Geometry check sheet. Reference: the model listing, model coordinates, mm. Face numbers are marked on the shaded views. A direction names the side the tool comes from. Coordinates: 2 decimals unless noted, no trailing zeros. Loops run counter-clockwise (first coordinate to the right, second up) from the corner with the lowest first, then second, coordinate; pieces in that order, holes last. Notation, with made-up numbers: (51, 73) - (100, 73) arc R36 cw to (100, 107) - close; hole circle Ø5 at (11, -7). An arc over 180 degrees is marked (long way). One line per item, written item: value.
from build123d import *

# Parameters (mm, degrees)
SKETCH1_R                    = 1.1303
BASE_DEPTH                   = 1.5
SKETCH1_4_W                  = 14.75
SKETCH1_4_H                  = 2
BOTTOM_WALLS_DEPTH           = 11
F_4_40_CLOSE_FIT_CLEAR_REACH = 41.1
SKETCH2_R                    = 1.4732
SKETCH1_8_W                  = 2
SKETCH1_8_H                  = 30.5
MIDDLE_WALLS_DEPTH           = 7
ROOF_START                   = 7
ROOF_OUTLINE_W               = 9.75
ROOF_OUTLINE_H               = 34.5
ROOF_DEPTH                   = 1
SKETCH1_5_W                  = 1.425
SKETCH1_5_H                  = 2.85
CUT_EXTRUDE2_DEPTH           = 8
FILLET1_R                    = 0.25


# Read off the part's stored shape, not the designer's step: Roof
with BuildPart() as part:
    # Sketch1 → Base (new body)
    with BuildSketch(Plane(origin=(0, 0, 0), x_dir=(1, 0, 0), z_dir=(0, 1, 0))):
        Polygon((5, -2), (14.75, -2), (14.75, 0), (0, 0), (0, -34.5), (14.75, -34.5), (14.75, -32.5), (5, -32.5), align=None)
        with Locations(Location((2.75, -7.25, 0), (0, 0, 270))):
            Circle(SKETCH1_R, mode=Mode.SUBTRACT)
        with Locations(Location((2.75, -27.25, 0), (0, 0, 270))):
            Circle(SKETCH1_R, mode=Mode.SUBTRACT)
    extrude(amount=BASE_DEPTH)

    # Sketch1<4> → Bottom Walls (add)
    with BuildSketch(Plane(origin=(0, 0, 0), x_dir=(1, 0, 0), z_dir=(0, 1, 0))):
        with Locations((7.375, -1)):
            Rectangle(SKETCH1_4_W, SKETCH1_4_H)
        with Locations((7.375, -33.5)):
            Rectangle(SKETCH1_4_W, SKETCH1_4_H)
    extrude(amount=-BOTTOM_WALLS_DEPTH)

    # 4-40_Close_fit Clear: up to this face of the body (flat: up to its plane)
    f_4_40_close_fit_clear_end = Plane(part.part.faces().sort_by_distance((7.375, -4.75, 0))[0])
    # Sketch2 → 4-40_Close_fit Clear (cut, up to the picked face)
    with BuildSketch(Plane.XY.offset(34.5), mode=Mode.PRIVATE) as f_4_40_close_fit_clear_sk1:
        with Locations((5.75, -7.58)):
            Circle(SKETCH2_R)
    f_4_40_close_fit_clear_tool1 = split(extrude(f_4_40_close_fit_clear_sk1.sketch, amount=-F_4_40_CLOSE_FIT_CLEAR_REACH, mode=Mode.PRIVATE), bisect_by=f_4_40_close_fit_clear_end, keep=Keep.BOTH, mode=Mode.PRIVATE)
    add(f_4_40_close_fit_clear_tool1.solids().sort_by(Axis((5.75, -7.58, 34.5), (0, 0, -1)))[0], mode=Mode.SUBTRACT)

    # Sketch1<8> → Middle Walls (add)
    with BuildSketch(Plane(origin=(0, 0, 0), x_dir=(1, 0, 0), z_dir=(0, 1, 0))):
        Polygon((5, -2), (7, -2), (12.75, -2), (14.75, -2), (14.75, 0), (5, 0), align=None)
        with Locations((6, -17.25)):
            Rectangle(SKETCH1_8_W, SKETCH1_8_H)
        Polygon((12.75, -32.5), (7, -32.5), (5, -32.5), (5, -34.5), (14.75, -34.5), (14.75, -32.5), align=None)
    extrude(amount=MIDDLE_WALLS_DEPTH)

    # Roof outline → Roof (add)
    with BuildSketch(Plane(origin=(0, 0, 0), x_dir=(1, 0, 0), z_dir=(0, 1, 0)).offset(ROOF_START)):
        with Locations((9.875, -17.25)):
            Rectangle(ROOF_OUTLINE_W, ROOF_OUTLINE_H)
    extrude(amount=ROOF_DEPTH)

    # Sketch1<5> → Cut-Extrude2 (cut)
    with BuildSketch(Plane(origin=(0, 0, 0), x_dir=(1, 0, 0), z_dir=(0, 1, 0))):
        with Locations((14.0375, -17.25)):
            Rectangle(SKETCH1_5_W, SKETCH1_5_H)
        with Locations((15.4625, -17.25)):
            Rectangle(SKETCH1_5_W, SKETCH1_5_H)
    extrude(amount=CUT_EXTRUDE2_DEPTH, mode=Mode.SUBTRACT)

    # Fillet1
    fillet1_edges = [part.edges().sort_by_distance(p)[0] for p in [
        (13.325, 7.5, 15.825),
        (13.325, 7.5, 18.675),
    ]]
    fillet(fillet1_edges, radius=FILLET1_R)


solid = part.part
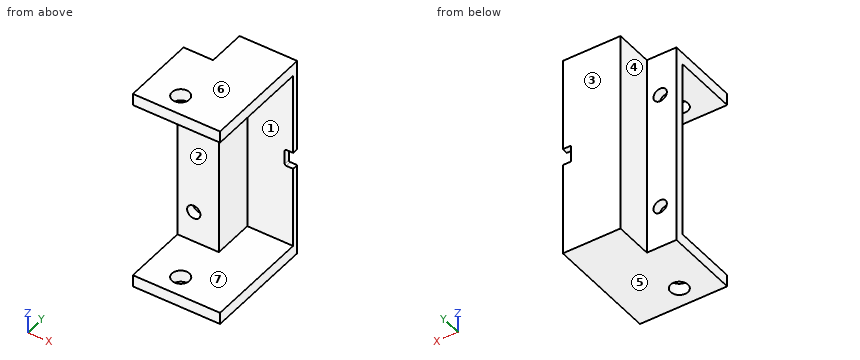
(1) Access from +Z, -Z, +X, -X, +Y, -Y to the whole of each face (thin tool, end or side, straight path). Record for the marked faces 1, 2, 3 and 4.
Reply:
face 1: +X, -Y
face 2: +X, -X, -Y
face 3: +Z, -Z, +X, -X, +Y
face 4: +Z, -Z, -X, +Y
(2) Go/stop test with flat-tipped pins: pin 1 Ø2 at (y, z) = (2, 12.5) entering from +X; pin 2 Ø2 at (x, z) = (4, 14.5) entering from -Y; pin 3 Ø1.5 at (x, z) = (3.5, 20) entering from +Y. Record where each tip stops, or that it passes through.
Reply:
pin 1: x = 7
pin 2: y = 0
pin 3: y = 1.5
(3) Cross-section at D-D on y = -7.58. Record the cut outline in (x, z), and give its area (3 significant figures).
Reply:
outline: (0, 0) - (4.28, 0) - (4.28, 2) - (0, 2) - close; (0, 32.5) - (4.28, 32.5) - (4.28, 34.5) - (0, 34.5) - close; (7.22, 0) - (14.75, 0) - (14.75, 2) - (7.22, 2) - close; (7.22, 32.5) - (14.75, 32.5) - (14.75, 34.5) - (7.22, 34.5) - close
area: 47.2 mm2
(4) Cross-section at B-B on x = 2.75. Record the cut outline in (y, z), and give its area (3 significant figures).
Reply:
outline: (-11, 0) - (1.5, 0) - (1.5, 6.12) - (0, 6.12) - (0, 2) - (-11, 2) - close; (-11, 32.5) - (0, 32.5) - (0, 28.38) - (1.5, 28.38) - (1.5, 34.5) - (-11, 34.5) - close; (0, 8.38) - (1.5, 8.38) - (1.5, 26.12) - (0, 26.12) - close
area: 89.0 mm2
(5) Cross-section at A-A on y = -1. Record the cut outline in (x, z).
Reply:
outline: (0, 0) - (14.75, 0) - (14.75, 2) - (0, 2) - close; (0, 32.5) - (14.75, 32.5) - (14.75, 34.5) - (0, 34.5) - close
(6) Release check for a two-part mould opening along Z. For the marked faces 5, 6 and 7 record: pulls with the +Z half, pulls with the -Z half, needs draft (parallel to the pull), parting line crosses it, or undercut.
Reply:
face 5: pulls with the -Z half
face 6: pulls with the +Z half
face 7: undercut
(7) Cross-section at C-C on z = 7.25. Record the cut outline in (x, y), and give its area (3 significant figures).
Reply:
outline: (0, 0) - (1.62, 0) - (1.62, 1.5) - (0, 1.5) - close; (3.88, 0) - (7, 0) - (7, 7) - (14.75, 7) - (14.75, 8) - (5, 8) - (5, 1.5) - (3.88, 1.5) - close
area: 27.9 mm2
(8) Material ranges on probe 1 along Y at (x, z) = (5.75, 0.75); probe 2 along Z at (x, y) = (10.75, -5.5); probe 3 along X at (y, z) = (0.8, 27.25), recorded low to high. Write a range as from..to.
Reply:
probe 1: -11..-9.05, -6.11..8
probe 2: 0..2, 32.5..34.5
probe 3: 0..1.62, 3.88..7
